Input: part model. Units: mm. Frame: model coordinates. Face numbers are marked on the shaded views. A direction names the side the tool comes from. Coordinates: 2 decimals unless noted, no trailing zeros. Write each loop counter-clockwise with the first axis right and the second up, starting at its lowest first coordinate (ties: lowest second). Pieces come first, ordered by that corner, then holes. Notation, with made-up numbers: (27, -13.75) - (83, -13.75) arc R14 ccw to (83, 4.25) - close; hole circle Ø1 at (28, 84). An arc over 180 degrees is marked (long way). Use CSV: the item, a comma, the result in double quotes.
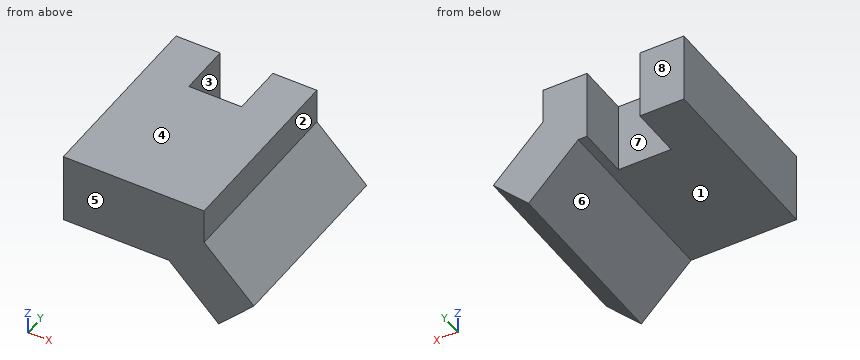
```python
from build123d import *

# Parameters (mm, degrees)
F1_DEPTH = 25.4
F2_SIZE  = 12.7
F3_DEPTH = 25.4


with BuildPart() as f1:
    # F0 (on Top) → F1 (new body)
    with BuildSketch(Plane.XY):
        Polygon((-25.4, -33.8918231428), (25.4, -33.8918231428), (25.4, 33.8918231428), (9.525, 33.8918231428), (9.525, 15.0958231428), (-9.525, 15.0958231428), (-9.525, 33.8918231428), (-25.4, 33.8918231428), align=None)
    extrude(amount=F1_DEPTH)

    # F2
    f2_edges = [f1.edges().sort_by_distance(p)[0] for p in [
        (25.4, 0, 0),
    ]]
    chamfer(f2_edges, length=F2_SIZE)

    # F3 (add): a face of the model
    f3_faces = [f1.faces().sort_by_distance(p)[0] for p in [
        (19.05, 0, 6.35),
    ]]
    extrude(f3_faces, amount=F3_DEPTH)


solid = f1.part
```
(1) Pin query (flat end, axial travel): pin 1 Ø15 at (y, z) = (27.5, 18.5) entering from +X; pin 2 Ø11.5 at (x, y) = (-4.5, 11) entering from -Z; pin 3 Ø21 at (x, z) = (-0.5, 13) entering from +Y; pin 4 Ø12 at (x, y) = (10, -9.5) entering from -Z. Return the tip coordinate at first contact, or that it passes through.
Check values:
pin 1,"x = 27.1"
pin 2,"z = 0"
pin 3,"y = 33.89"
pin 4,"z = -3.3"
(2) Cut plane B-B on y = 1. Return loops of the section in (x, z), and give its area (3 significant figures).
Check values:
outline,"(-25.4, 0) - (12.7, 0) - (30.66, -17.96) - (43.36, -5.26) - (25.4, 12.7) - (25.4, 25.4) - (-25.4, 25.4) - close"
area,"1,670 mm^2"
(3) Reachability of the marked faces 1, 2, 3, 4 and 5 from +Z, -Z, +X, -X, +Y, -Y: full face, straight path, thin tool, end or side. Return the list, or none.
Check values:
face 1,"-Z, -X, +Y, -Y"
face 2,"+Z, +X, +Y, -Y"
face 3,"+Z, -Z, +Y"
face 4,"+Z, +X, -X, +Y, -Y"
face 5,"+Z, -Z, +X, -X, -Y"
(4) Cut plane A-A on z = 10. Return loops of the section in (x, y) (3 decimals).
Check values:
outline,"(-25.4, -33.892) - (28.1, -33.892) - (28.1, 33.892) - (9.525, 33.892) - (9.525, 15.096) - (-9.525, 15.096) - (-9.525, 33.892) - (-25.4, 33.892) - close"
(5) Cut plane D-D on z = 22. Return loops of the section in (x, y) (3 decimals).
Check values:
outline,"(-25.4, -33.892) - (25.4, -33.892) - (25.4, 33.892) - (9.525, 33.892) - (9.525, 15.096) - (-9.525, 15.096) - (-9.525, 33.892) - (-25.4, 33.892) - close"
(6) Draft query along X for the marked faces 6, 7 and 8. Return one class per face: pulls with the +X half, pulls with the -X half, needs draft (parallel to the pull), parting line crosses it, or undercut.
Check values:
face 6,"pulls with the -X half"
face 7,"undercut"
face 8,"needs draft"
(7) Ray query, probe 1 along X at (y, z) = (18, 20.5) (3 decimals); probe 2 along X at (y, z) = (8, 17); probe 3 along Z at (x, y) = (5, 10). Return the intervals inside material, ascending. Write a range as from..to.
Check values:
probe 1,"-25.4..-9.525, 9.525..25.4"
probe 2,"-25.4..25.4"
probe 3,"0..25.4"
(8) Cut plane C-C on x = 15. Return loops of the section in (y, z), and give its area (3 significant figures).
Check values:
outline,"(-33.89, -2.3) - (33.89, -2.3) - (33.89, 25.4) - (-33.89, 25.4) - close"
area,"1,880 mm^2"
